from build123d import *

# Parameters (mm, degrees)
EXTRUDE_1_DEPTH     = 1000
CUT_EXTRUDE_3_DEPTH = 1003.594743762
CUT_EXTRUDE_5_DEPTH = 1003.62092087


with BuildPart() as part:
    # 草图1 → 凸台-拉伸1 (new body)
    with BuildSketch(Plane(origin=(0, 0, 0), x_dir=(0, 0, -1), z_dir=(1, 0, 0))):
        with BuildLine():
            Line((-0.5, 0), (-45.41834413, 0))
            ThreePointArc((-45.41834413, 0), (-48.796295168, 1.313613316), (-50.39931762, 4.564221286))
            Line((-50.39931762, 4.564221286), (-54.314209266, 49.311637556))
            ThreePointArc((-54.314209266, 49.311637556), (-54.199134139, 49.676609232), (-53.859689788, 49.853312776))
            Line((-53.859689788, 49.853312776), (-52.86349509, 49.940468519))
            ThreePointArc((-52.86349509, 49.940468519), (-52.498523414, 49.825393391), (-52.32181987, 49.485949041))
            Line((-52.32181987, 49.485949041), (-48.406928224, 4.738532772))
            ThreePointArc((-48.406928224, 4.738532772), (-47.445114753, 2.78816799), (-45.41834413, 2))
            Line((-45.41834413, 2), (-0.5, 2))
            ThreePointArc((-0.5, 2), (-0.146446609, 1.853553391), (0, 1.5))
            Line((0, 1.5), (0, 0.5))
            ThreePointArc((0, 0.5), (-0.146446609, 0.146446609), (-0.5, 0))
        make_face()
    extrude(amount=EXTRUDE_1_DEPTH)

    # 草图3 → 切除-拉伸3 (cut, through all)
    with BuildSketch(Plane(origin=(0, -4.166892956, 47.627804429), x_dir=(-1, 0, 0), z_dir=(0, 0.08715574274765506, -0.9961946980917459))):
        with BuildLine():
            Line((-59.5, 40.939443007), (-24.5, 40.939443007))
            ThreePointArc((-24.5, 40.939443007), (-15.5, 31.939443007), (-24.5, 22.939443007))
            Line((-24.5, 22.939443007), (-59.5, 22.939443007))
            ThreePointArc((-59.5, 22.939443007), (-68.5, 31.939443007), (-59.5, 40.939443007))
        make_face()
        with BuildLine():
            Line((-129.5, 40.939443007), (-94.5, 40.939443007))
            ThreePointArc((-94.5, 40.939443007), (-85.5, 31.939443007), (-94.5, 22.939443007))
            Line((-94.5, 22.939443007), (-129.5, 22.939443007))
            ThreePointArc((-129.5, 22.939443007), (-138.5, 31.939443007), (-129.5, 40.939443007))
        make_face()
        with BuildLine():
            Line((-199.5, 40.939443007), (-164.5, 40.939443007))
            ThreePointArc((-164.5, 40.939443007), (-155.5, 31.939443007), (-164.5, 22.939443007))
            Line((-164.5, 22.939443007), (-199.5, 22.939443007))
            ThreePointArc((-199.5, 22.939443007), (-208.5, 31.939443007), (-199.5, 40.939443007))
        make_face()
        with BuildLine():
            Line((-269.5, 40.939443007), (-234.5, 40.939443007))
            ThreePointArc((-234.5, 40.939443007), (-225.5, 31.939443007), (-234.5, 22.939443007))
            Line((-234.5, 22.939443007), (-269.5, 22.939443007))
            ThreePointArc((-269.5, 22.939443007), (-278.5, 31.939443007), (-269.5, 40.939443007))
        make_face()
        with BuildLine():
            Line((-339.5, 40.939443007), (-304.5, 40.939443007))
            ThreePointArc((-304.5, 40.939443007), (-295.5, 31.939443007), (-304.5, 22.939443007))
            Line((-304.5, 22.939443007), (-339.5, 22.939443007))
            ThreePointArc((-339.5, 22.939443007), (-348.5, 31.939443007), (-339.5, 40.939443007))
        make_face()
        with BuildLine():
            Line((-409.5, 40.939443007), (-374.5, 40.939443007))
            ThreePointArc((-374.5, 40.939443007), (-365.5, 31.939443007), (-374.5, 22.939443007))
            Line((-374.5, 22.939443007), (-409.5, 22.939443007))
            ThreePointArc((-409.5, 22.939443007), (-418.5, 31.939443007), (-409.5, 40.939443007))
        make_face()
        with BuildLine():
            Line((-479.5, 40.939443007), (-444.5, 40.939443007))
            ThreePointArc((-444.5, 40.939443007), (-435.5, 31.939443007), (-444.5, 22.939443007))
            Line((-444.5, 22.939443007), (-479.5, 22.939443007))
            ThreePointArc((-479.5, 22.939443007), (-488.5, 31.939443007), (-479.5, 40.939443007))
        make_face()
        with BuildLine():
            Line((-549.5, 40.939443007), (-514.5, 40.939443007))
            ThreePointArc((-514.5, 40.939443007), (-505.5, 31.939443007), (-514.5, 22.939443007))
            Line((-514.5, 22.939443007), (-549.5, 22.939443007))
            ThreePointArc((-549.5, 22.939443007), (-558.5, 31.939443007), (-549.5, 40.939443007))
        make_face()
        with BuildLine():
            Line((-619.5, 40.939443007), (-584.5, 40.939443007))
            ThreePointArc((-584.5, 40.939443007), (-575.5, 31.939443007), (-584.5, 22.939443007))
            Line((-584.5, 22.939443007), (-619.5, 22.939443007))
            ThreePointArc((-619.5, 22.939443007), (-628.5, 31.939443007), (-619.5, 40.939443007))
        make_face()
        with BuildLine():
            Line((-689.5, 40.939443007), (-654.5, 40.939443007))
            ThreePointArc((-654.5, 40.939443007), (-645.5, 31.939443007), (-654.5, 22.939443007))
            Line((-654.5, 22.939443007), (-689.5, 22.939443007))
            ThreePointArc((-689.5, 22.939443007), (-698.5, 31.939443007), (-689.5, 40.939443007))
        make_face()
        with BuildLine():
            Line((-759.5, 40.939443007), (-724.5, 40.939443007))
            ThreePointArc((-724.5, 40.939443007), (-715.5, 31.939443007), (-724.5, 22.939443007))
            Line((-724.5, 22.939443007), (-759.5, 22.939443007))
            ThreePointArc((-759.5, 22.939443007), (-768.5, 31.939443007), (-759.5, 40.939443007))
        make_face()
        with BuildLine():
            Line((-829.5, 40.939443007), (-794.5, 40.939443007))
            ThreePointArc((-794.5, 40.939443007), (-785.5, 31.939443007), (-794.5, 22.939443007))
            Line((-794.5, 22.939443007), (-829.5, 22.939443007))
            ThreePointArc((-829.5, 22.939443007), (-838.5, 31.939443007), (-829.5, 40.939443007))
        make_face()
        with BuildLine():
            Line((-899.5, 40.939443007), (-864.5, 40.939443007))
            ThreePointArc((-864.5, 40.939443007), (-855.5, 31.939443007), (-864.5, 22.939443007))
            Line((-864.5, 22.939443007), (-899.5, 22.939443007))
            ThreePointArc((-899.5, 22.939443007), (-908.5, 31.939443007), (-899.5, 40.939443007))
        make_face()
        with BuildLine():
            Line((-969.5, 40.939443007), (-934.5, 40.939443007))
            ThreePointArc((-934.5, 40.939443007), (-925.5, 31.939443007), (-934.5, 22.939443007))
            Line((-934.5, 22.939443007), (-969.5, 22.939443007))
            ThreePointArc((-969.5, 22.939443007), (-978.5, 31.939443007), (-969.5, 40.939443007))
        make_face()
    extrude(amount=-CUT_EXTRUDE_3_DEPTH, mode=Mode.SUBTRACT)

    # 草图2 → 切除-拉伸5 (cut, through all)
    with BuildSketch(Plane(origin=(0, 2, 0), x_dir=(1, 0, 0), z_dir=(0, 1, 0))):
        with BuildLine():
            Line((59.5, -14.5), (24.5, -14.5))
            ThreePointArc((24.5, -14.5), (15.5, -23.5), (24.5, -32.5))
            Line((24.5, -32.5), (59.5, -32.5))
            ThreePointArc((59.5, -32.5), (68.5, -23.5), (59.5, -14.5))
        make_face()
        with BuildLine():
            Line((129.5, -14.5), (94.5, -14.5))
            ThreePointArc((94.5, -14.5), (85.5, -23.5), (94.5, -32.5))
            Line((94.5, -32.5), (129.5, -32.5))
            ThreePointArc((129.5, -32.5), (138.5, -23.5), (129.5, -14.5))
        make_face()
        with BuildLine():
            Line((199.5, -14.5), (164.5, -14.5))
            ThreePointArc((164.5, -14.5), (155.5, -23.5), (164.5, -32.5))
            Line((164.5, -32.5), (199.5, -32.5))
            ThreePointArc((199.5, -32.5), (208.5, -23.5), (199.5, -14.5))
        make_face()
        with BuildLine():
            Line((269.5, -14.5), (234.5, -14.5))
            ThreePointArc((234.5, -14.5), (225.5, -23.5), (234.5, -32.5))
            Line((234.5, -32.5), (269.5, -32.5))
            ThreePointArc((269.5, -32.5), (278.5, -23.5), (269.5, -14.5))
        make_face()
        with BuildLine():
            Line((339.5, -14.5), (304.5, -14.5))
            ThreePointArc((304.5, -14.5), (295.5, -23.5), (304.5, -32.5))
            Line((304.5, -32.5), (339.5, -32.5))
            ThreePointArc((339.5, -32.5), (348.5, -23.5), (339.5, -14.5))
        make_face()
        with BuildLine():
            Line((409.5, -14.5), (374.5, -14.5))
            ThreePointArc((374.5, -14.5), (365.5, -23.5), (374.5, -32.5))
            Line((374.5, -32.5), (409.5, -32.5))
            ThreePointArc((409.5, -32.5), (418.5, -23.5), (409.5, -14.5))
        make_face()
        with BuildLine():
            Line((479.5, -14.5), (444.5, -14.5))
            ThreePointArc((444.5, -14.5), (435.5, -23.5), (444.5, -32.5))
            Line((444.5, -32.5), (479.5, -32.5))
            ThreePointArc((479.5, -32.5), (488.5, -23.5), (479.5, -14.5))
        make_face()
        with BuildLine():
            Line((549.5, -14.5), (514.5, -14.5))
            ThreePointArc((514.5, -14.5), (505.5, -23.5), (514.5, -32.5))
            Line((514.5, -32.5), (549.5, -32.5))
            ThreePointArc((549.5, -32.5), (558.5, -23.5), (549.5, -14.5))
        make_face()
        with BuildLine():
            Line((619.5, -14.5), (584.5, -14.5))
            ThreePointArc((584.5, -14.5), (575.5, -23.5), (584.5, -32.5))
            Line((584.5, -32.5), (619.5, -32.5))
            ThreePointArc((619.5, -32.5), (628.5, -23.5), (619.5, -14.5))
        make_face()
        with BuildLine():
            Line((689.5, -14.5), (654.5, -14.5))
            ThreePointArc((654.5, -14.5), (645.5, -23.5), (654.5, -32.5))
            Line((654.5, -32.5), (689.5, -32.5))
            ThreePointArc((689.5, -32.5), (698.5, -23.5), (689.5, -14.5))
        make_face()
        with BuildLine():
            Line((759.5, -14.5), (724.5, -14.5))
            ThreePointArc((724.5, -14.5), (715.5, -23.5), (724.5, -32.5))
            Line((724.5, -32.5), (759.5, -32.5))
            ThreePointArc((759.5, -32.5), (768.5, -23.5), (759.5, -14.5))
        make_face()
        with BuildLine():
            Line((829.5, -14.5), (794.5, -14.5))
            ThreePointArc((794.5, -14.5), (785.5, -23.5), (794.5, -32.5))
            Line((794.5, -32.5), (829.5, -32.5))
            ThreePointArc((829.5, -32.5), (838.5, -23.5), (829.5, -14.5))
        make_face()
        with BuildLine():
            Line((899.5, -14.5), (864.5, -14.5))
            ThreePointArc((864.5, -14.5), (855.5, -23.5), (864.5, -32.5))
            Line((864.5, -32.5), (899.5, -32.5))
            ThreePointArc((899.5, -32.5), (908.5, -23.5), (899.5, -14.5))
        make_face()
        with BuildLine():
            Line((969.5, -14.5), (934.5, -14.5))
            ThreePointArc((934.5, -14.5), (925.5, -23.5), (934.5, -32.5))
            Line((934.5, -32.5), (969.5, -32.5))
            ThreePointArc((969.5, -32.5), (978.5, -23.5), (969.5, -14.5))
        make_face()
    extrude(amount=-CUT_EXTRUDE_5_DEPTH, mode=Mode.SUBTRACT)


solid = part.part
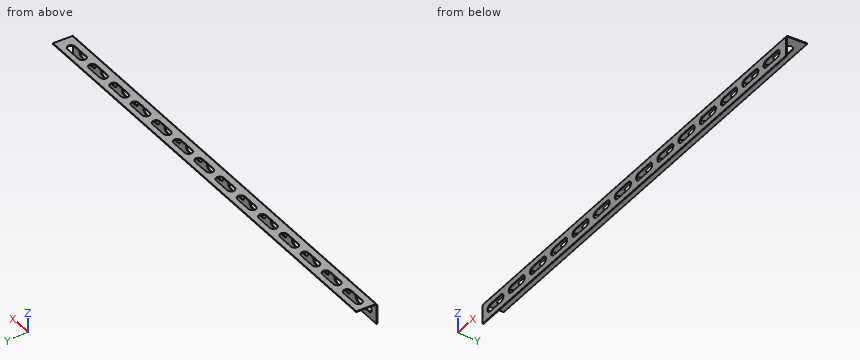
Source: CAD feature listing. Evaluate the final solid. Frame: model axes, mm. Give positions to 0.01 mm unless a question says otherwise; leave off trailing zeros. Write each loop counter-clockwise with the first axis right and the second up, starting at its lowest first coordinate (ties: lowest second). Pieces come first, ordered by that corner, then holes. Notation, with made-up numbers: M -9,89 L 38,89 A19 cw 38,118 Z; hole C 84,24 d10. An arc over 180 degrees is marked long. Answer as a JSON object with one key per item and string values.
Q1. Contact query for flat-ended pins moving along their axis: P1, Ø3, axis at x = 702, z = 10, coming from the +Y side; P2, Ø1, axis at x = 117, y = 1.5, coming from the +Z side; P3, Ø0.6, axis at x = 748, y = 1.5, coming from the +Z side; P4, Ø1.5, axis at x = 723.5, z = 31.5, coming from the -Y side. Output: stop coordinate, or through.
Geometry check:
{"P1": "stops at y = 2", "P2": "stops at z = 49.42", "P3": "stops at z = 49.26", "P4": "passes through"}
Q2. Cut plane B-B, the plane z = 23.5. Count the separate pieces of the cut face and the enclosed holes in it, then the cut area to 3 significant figures.
Geometry check:
{"separate pieces": "15", "enclosed holes": "0", "area": "516 mm^2"}
Q3. Cut plane A-A, the plane x = 742. Return the cut outline in (y, z), then the cut area to 3 significant figures.
Geometry check:
{"outline": "M 0,0.5 A0.5 ccw 0.5,0 L 1.5,0 A0.5 ccw 2,0.5 L 2,14.5 L 0,14.5 Z; M 0,32.5 L 2,32.5 L 2,45.42 A3 cw 4.74,48.41 L 18.69,49.63 L 18.51,51.62 L 4.56,50.4 A5 ccw 0,45.42 Z; M 36.44,53.19 L 36.62,51.2 L 49.49,52.32 A0.5 ccw 49.94,52.86 L 49.85,53.86 A0.5 ccw 49.31,54.31 Z", "area": "121 mm^2"}
Q4. Ray query, line 1 along Z through (x, y) = (512, 37); line 2 along Y through (x, z) = (648, 11); line 3 along Z through (x, y) = (454, 5.5). Return the intervals inside material, ascending.
Geometry check:
{"line 1": "z = 51.23 to 53.24", "line 2": "y = 0 to 2", "line 3": "z = 48.47 to 50.48"}
